```python
from build123d import *

# Parameters (mm, degrees)
F1_DEPTH = 25.4
F2_R     = 6.35
F3_DEPTH = 25.4
F4_R     = 6.35
F5_DEPTH = 12.7
F7_DEPTH = 12.7


# Not quite as in the source:
# - ends of sketch curves that miss each other by under 0.0002 mm in the source are joined


with BuildPart() as f1:
    # F0 (on Front) → F1 (new body)
    with BuildSketch(Plane.XZ):
        Polygon((0, 12.7), (0, 0), (76.2, 0), (76.2, 12.7), (50.8, 12.7), (50.8, 44.45), (25.4, 44.45), (25.4, 12.7), align=None)
    extrude(amount=F1_DEPTH)

    # F2 (on face) → F3 (cut)
    with BuildSketch(Plane.YZ.offset(50.8)):
        with Locations((-12.7, 31.75)):
            Circle(F2_R)
        with BuildLine():
            ThreePointArc((-12.6538738539, 44.4500834572), (-4.2011824857, 41.2444061447), (0, 33.2397559887))
            Line((0, 33.2397559887), (0, 44.45))
            Line((0, 44.45), (-12.6538738539, 44.4500834572))
        make_face()
        with BuildLine():
            ThreePointArc((-25.4, 31.8358913064), (-21.6202217079, 40.7633957722), (-12.6538738539, 44.4500834572))
            Line((-12.6538738539, 44.4500834572), (-25.4, 44.45))
            Line((-25.4, 44.45), (-25.4, 31.8358913064))
        make_face()
    extrude(amount=-F3_DEPTH, mode=Mode.SUBTRACT)

    # F4 (on face) → F5 (cut)
    with BuildSketch(Plane.XY.offset(12.7)):
        with Locations((12.7003350629, -12.6999999956)):
            Circle(F4_R)
        with BuildLine():
            ThreePointArc((0, -12.7), (3.7197438789, -3.7197438789), (12.7, 0))
            Line((12.7, 0), (0, 0))
            Line((0, 0), (0, -12.7))
        make_face()
        with Locations((63.5, -12.7)):
            Circle(F4_R)
        with BuildLine():
            Line((0, -25.4), (12.7, -25.4))
            ThreePointArc((12.7, -25.4), (3.7197438789, -21.6802561211), (0, -12.7))
            Line((0, -12.7), (0, -25.4))
        make_face()
    extrude(amount=-F5_DEPTH, mode=Mode.SUBTRACT)

    # F6 (on face) → F7 (cut)
    with BuildSketch(Plane.XY.offset(12.7)):
        with BuildLine():
            ThreePointArc((76.2000025586, -12.7), (72.4802576974, -21.6802565734), (63.5, -25.3999987207))
            Line((63.5, -25.3999987207), (76.2, -25.4))
            Line((76.2, -25.4), (76.2000025586, -12.7))
        make_face()
        with BuildLine():
            ThreePointArc((63.5, -1.2793e-06), (72.4802576975, -3.7197434266), (76.2000025586, -12.7))
            Line((76.2000025586, -12.7), (76.2, 0))
            Line((76.2, 0), (63.5, -1.2793e-06))
        make_face()
    extrude(amount=-F7_DEPTH, mode=Mode.SUBTRACT)


solid = f1.part
```
Geometry: final body of the model. Coordinates: model frame, mm. A direction names the side the tool comes from. Coordinates: 2 decimals unless noted, no trailing zeros. Write each loop counter-clockwise with the first axis right and the second up, starting at its lowest first coordinate (ties: lowest second). Pieces come first, ordered by that corner, then holes. Notation, with made-up numbers: M 59,42.5 L 73,42.5 A10 ccw 73,61.5 Z; hole C 46,-11 d10. An arc over 180 degrees is marked long. Answer as CSV lines item,"result". Start each with the question number.
Q1. Cut plane A-A on x = 34.5. Return the cut outline in (y, z), then the cut area to 3 significant figures.
Q2. Cut plane C-C on y = -2.75. Return the cut outline in (x, z), then the cut area to 3 significant figures.
Q3. Mould query, pull axis X, two halves, no side actions, for faces 4 (the cylindrical face through (18.566, -15.132, 6.439)), 5 (the flat face through (55, -13, 12.7)), 6 (the cylindrical face through (72.38, -3.62, 6.44)), 7 (the cylindrical face through (62.12, -18.9, 6.44)). Classes: released by +X, released by -X, zero draft, split by the parting line, or undercut.
Q4. Pin query (flat end, axial travel): P1, Ø11.5, axis at x = 63.5, y = -12.7, coming from the -Z side; P2, Ø8, axis at y = -16.5, z = 14.5, coming from the +X side; P3, Ø8, axis at y = -19, z = 39, coming from the +X side; P4, Ø5, axis at x = 24, y = -8, coming from the +Z side. Return the tip coordinate at first contact, or that it passes through.
Q5. Reachability of faces 1 (the flat face through (38, 0, 13)), 2 (the flat face through (25.4, -13, 25)), 3 (the flat face through (50.8, -13, 25)) from +Z, -Z, +X, -X, +Y, -Y: full face, straight path, thin tool, end or side. Return the list, or none.
Q6. Cut plane B-B on z = 29.5. Return the cut outline in (x, y), then the cut area to 3 significant figures.
Q7. Cut plane D-D on x = 58. Return the cut outline in (y, z).
Q8. Line query: line 1 (Z direction, x = 7, y = -3.5); line 2 (Y direction, x = 28, z = 32.5); line 3 (X direction, y = -7.5, z = 24). Output: solid intervals per line, ascending. Write a range as from..to.
Findings below:
1,outline,"M -25.4,0 L 0,0 L 0,33.24 A12.75 ccw -12.61,44.45 L -12.7,44.45 A12.75 ccw -25.4,31.84 Z; hole C -12.7,31.75 d12.7"
1,area,"934 mm2"
2,outline,"M 4.81,0 L 71.39,0 L 71.39,12.7 L 50.8,12.7 L 50.8,39.73 L 25.4,39.73 L 25.4,12.7 L 4.81,12.7 Z"
2,area,"1,530 mm2"
3,face 4,"undercut"
3,face 5,"zero draft"
3,face 6,"released by +X"
3,face 7,"undercut"
4,P1,"passes through"
4,P2,"stops at x = 76.2"
4,P3,"stops at x = 50.8"
4,P4,"stops at z = 44.19"
5,face 1,"+Z, -Z, +X, -X, +Y"
5,face 2,"+Z, -X, +Y, -Y"
5,face 3,"+Z, +X, +Y, -Y"
6,outline,"M 25.4,-25.4 L 50.8,-25.4 L 50.8,-18.64 L 25.4,-18.64 Z; M 25.4,-6.76 L 50.8,-6.76 L 50.8,0 L 25.4,0 Z"
6,area,"344 mm2"
7,outline,"M -25.4,0 L -15.87,0 L -15.87,12.7 L -25.4,12.7 Z; M -9.53,0 L 0,0 L 0,12.7 L -9.53,12.7 Z"
8,line 1,"z = 0..12.7"
8,line 2,"y = -25.38..-19.01, -6.39..0"
8,line 3,"x = 25.4..50.8"
